from build123d import *

# Parameters (mm, degrees)
F0_R     = 15.875
F1_DEPTH = 4.191
F3_D     = 3.4544
F3_DEPTH = 14.2875
F3_TIP   = 1.0378064612


with BuildPart() as f1:
    # F0 (on Front) → F1 (new body, symmetric)
    with BuildSketch(Plane.XZ):
        with BuildLine():
            ThreePointArc((-17.1823825283, -9.8631168831), (19.812, 0), (-17.1823825283, 9.8631168831))
            ThreePointArc((-17.1823825283, 9.8631168831), (-20.6703460499, 6.362061759), (-25.4431433593, 5.08))
            Line((-25.4431433593, 5.08), (-31.7931433593, 5.08))
            Line((-31.7931433593, 5.08), (-31.7931433593, -5.08))
            Line((-31.7931433593, -5.08), (-25.4431433593, -5.08))
            ThreePointArc((-25.4431433593, -5.08), (-20.6703460499, -6.362061759), (-17.1823825283, -9.8631168831))
        make_face()
        Circle(F0_R, mode=Mode.SUBTRACT)
    extrude(amount=F1_DEPTH, both=True)

    # F3
    with Locations(Plane(origin=(-31.7931433593, 0, 0), x_dir=(0, -1, 0), z_dir=(-1, 0, 0))):
        with Locations((0, 0)):
            Hole(F3_D / 2, depth=F3_DEPTH)
            with Locations((0, 0, -(F3_DEPTH + F3_TIP / 2))):  # 118° drill point
                Cone(0, F3_D / 2, F3_TIP, mode=Mode.SUBTRACT)


solid = f1.part
Design review of the part built by this model. Coordinates are the model's own, in mm. A direction names the side the tool comes from. Round coordinates to 2 decimals unless told otherwise and drop trailing zeros. Order: outer loops, then holes, each group sorted by start corner. A loop starts at its lowest first (then second) coordinate and runs counter-clockwise, first axis right, second up.
1) Draft analysis for pull direction Z (two halves, no side actions). For faces 1 (the cylindrical face through (-20.73, -0.06, -6.33)), 2 (the conical face through (-16.65, -0.28, -0.11)), 3 (the flat face through (-29, 0, 5.08)), state which applies: released by +Z, released by -Z, zero draft, split by the parting line, or undercut.
The answers:
face 1: released by -Z
face 2: undercut
face 3: released by +Z
2) Clearance check with flat-ended pins moving along their axes: pin 1 Ø3 at (y, z) = (-2.5, -11) entering from +X; pin 2 Ø3 at (y, z) = (0, 0) entering from -X; pin 3 Ø3 at (y, z) = (1, 8) entering from -X. State where each tip first meets the part, or that it passes through.
The answers:
pin 1: stops at x = 17.39
pin 2: stops at x = -17.37
pin 3: stops at x = -20.44
3) For L1, parallel to Z at x = 0, y = 2 (3 decimals); L2, parallel to Y at x = -25.5, z = 0; L3, parallel to X at y = 2.75, z = 11, list the stretches that pass through material, from the lowest coordinate up.
The answers:
L1: z = -19.812 to -15.875, 15.875 to 19.812
L2: y = -4.19 to -1.73, 1.73 to 4.19
L3: x = -16.48 to -11.45, 11.45 to 16.48
4) Machinability: for faces 4 (the cylindrical face through (-24.549, -0.225, 1.713)), 5 (the cylindrical face through (-20.61, -0.059, 6.397)), 6 (the flat face through (-29, 0, -5.08)), which of the approach directions +Z, -Z, +X, -X, +Y, -Y give a long, thin tool a straight path to every point of the face, cutting with its end or side? Answer none if there is none.
The answers:
face 4: -X
face 5: +Z, -X, +Y, -Y
face 6: -Z, -X, +Y, -Y
5) Consider section A-A (x = 0). State the section outline as (y, z) points (3 decimals), plus the area to 3 significant figures.
The answers:
outline: (-4.191, -19.812) - (4.191, -19.812) - (4.191, -15.875) - (-4.191, -15.875) - close; (-4.191, 15.875) - (4.191, 15.875) - (4.191, 19.812) - (-4.191, 19.812) - close
area: 66.0 mm2
6) Consider section B-B (z = -6.5). State the section outline as (x, y) points, plus the area to 3 significant figures.
The answers:
outline: (-20.44, -4.19) - (-14.48, -4.19) - (-14.48, 4.19) - (-20.44, 4.19) - close; (14.48, -4.19) - (18.72, -4.19) - (18.72, 4.19) - (14.48, 4.19) - close
area: 85.4 mm2
